Design review of the part built by this model. Coordinates are the model's own, in mm. Coordinates: 2 decimals unless noted, no trailing zeros. Write each loop counter-clockwise with the first axis right and the second up, starting at its lowest first coordinate (ties: lowest second). Pieces come first, ordered by that corner, then holes.
Autodesk Inventor part; units mm, degrees
ref_plane "YZ Plane" through (0, 0, 0) normal (1, 0, 0) x (0, 1, 0)
ref_plane "XZ Plane" through (0, 0, 0) normal (0, 1, 0) x (-1, 0, 0)
ref_plane "XY Plane" through (0, 0, 0) normal (0, 0, 1) x (1, 0, 0)
sketch "Sketch1" plane through (0, 0, 0) normal (0, 0, 1) x (1, 0, 0)
  line L0 (40, 4.4544) -> (40, 94.4544)
  line L1 (40, 94.4544) -> (0, 94.4544)
  line L2 (0, 94.4544) -> (0, 4.4544)
  circle A0 centre (20, 59.4544) radius 4.25
  circle A1 centre (10, 14.4544) radius 2.1
  circle A2 centre (30, 14.4544) radius 2.1
  circle A3 centre (19.982, 77.4544) radius 2.5
  circle A4 centre (19.8755, 41.4544) radius 2.5
  line L3 (0, 4.4544) -> (40, 4.4544)
  point P0 (0, 0)
  dimension "d4" = 40
  dimension "d5" = 90
  dimension "d7" = 8.5
  dimension "d8" = 35
  dimension "d9" = 20
  dimension "d11" = 90
  dimension "d19" = 10
  dimension "d21" = 4.2
  dimension "d22" = 10
  dimension "d24" = 4.2
extrude "Extrusion1" add sketch "Sketch1" along normal blind 6
fillet "Fillet1" radius 5 2 edges at (0, 94.4544, 3) (40, 94.4544, 3)
equation "\"d9\" = 0.5 * d4"
equation "\"d24\" = d21"
properties part number "BaseC_5" material "PMMA Plastic"
(1) Consider section C-C (z = 3.15). Give the boundary of the cut face in (x, y).
(2) Consider section B-B (x = 20). Give the boundary of the cut face in (y, z), plus the area to 3 significant figures.
(3) Wall thickness on line 1 (Y direction, x = 20, z = 1.45); line 2 (X direction, y = 59.5, z = 5.6); line 3 (Y direction, x = 22, z = 3.6): over which ranges is each line inside the solid? List them lowest first.
(4) Consider section A-A (x = 10). Give the boundary of the cut face in (y, z), plus the area to 3 significant figures.
(5) Mouldability with a two-part tool opening along Y and no side actions: class faces 1 (the flat face through (20, 50, 0)), 2 (the cylindrical face through (38.574, 92.951, 3.042)), 3 (the cylindrical face through (7.9, 14.4, 3)) as +Y half, -Y half, draft (parallel to the pull), parting line (faces both ways), or undercut.
(6) Insertion check: pin 1 Ø4 at (x, y) = (19.88, 41.45) entering from +Z; pin 2 Ø2 at (x, y) = (31, 70) entering from -Z. Each pin has a flat end and moves straight along its axis. Give the tip position at first contact, or say it passes through.
Results:
1. outline: (0, 4.45) - (40, 4.45) - (40, 89.45) arc R5 ccw to (35, 94.45) - (5, 94.45) arc R5 ccw to (0, 89.45) - close; hole circle Ø4.2 at (10, 14.45); hole circle Ø8.5 at (20, 59.45); hole circle Ø5 at (19.88, 41.45); hole circle Ø5 at (19.98, 77.45); hole circle Ø4.2 at (30, 14.45)
2. outline: (4.45, 0) - (38.96, 0) - (38.96, 6) - (4.45, 6) - close; (43.95, 0) - (55.2, 0) - (55.2, 6) - (43.95, 6) - close; (63.7, 0) - (74.95, 0) - (74.95, 6) - (63.7, 6) - close; (79.95, 0) - (94.45, 0) - (94.45, 6) - (79.95, 6) - close
2. area: 429 mm2
3. line 1: y = 4.45 to 38.96, 43.95 to 55.2, 63.7 to 74.95, 79.95 to 94.45
3. line 2: x = 0 to 15.75, 24.25 to 40
3. line 3: y = 4.45 to 40.14, 42.77 to 55.7, 63.2 to 75.98, 78.93 to 94.45
4. outline: (4.45, 0) - (12.35, 0) - (12.35, 6) - (4.45, 6) - close; (16.55, 0) - (94.45, 0) - (94.45, 6) - (16.55, 6) - close
4. area: 515 mm2
5. face 1: draft
5. face 2: +Y half
5. face 3: undercut
6. pin 1: passes through
6. pin 2: stops at z = 0
